For this review, take the finished solid that the model builds, in its own axes (mm). A direction names the side the tool comes from. Round coordinates to 2 decimals unless told otherwise and drop trailing zeros. Order: outer loops, then holes, each group sorted by start corner. A loop starts at its lowest first (then second) coordinate and runs counter-clockwise, first axis right, second up. Notation, with made-up numbers: M 78.5,9 L 119.5,9 A33 ccw 119.5,42 Z; hole C 17,46 d4. An arc over 180 degrees is marked long. Answer as a JSON object with one key per item and string values.
from build123d import *

# Parameters (mm, degrees)
AUFSATZ_LINEAR_AUSTRAGEN2_DEPTH = 14
SKIZZE3_W                       = 10.8
SKIZZE3_H                       = 4
SKIZZE3_H_2                     = 8
SCHNITT_LINEAR_AUSTRAGEN1_DEPTH = 201.389926144
SCHNITT_LINEAR_AUSTRAGEN2_DEPTH = 202.674849696


with BuildPart() as part:
    # Skizze1 → Aufsatz-Linear austragen2 (new, symmetric)
    with BuildSketch(Plane.XY):
        with BuildLine():
            Line((-198.15, 0), (-198.15, -2))
            Line((-198.15, -2), (-199.65, -2))
            Line((-199.65, -2), (-199.65, 0))
            ThreePointArc((-199.65, 0), (-198.288046533, 3.288046533), (-195, 4.65))
            Line((-195, 4.65), (195, 4.65))
            ThreePointArc((195, 4.65), (198.288046533, 3.288046533), (199.65, 0))
            Line((199.65, 0), (199.65, -2))
            Line((199.65, -2), (198.15, -2))
            Line((198.15, -2), (198.15, 0))
            ThreePointArc((198.15, 0), (195, 3.15), (191.85, 0))
            Line((191.85, 0), (191.85, -2))
            Line((191.85, -2), (188.85, -2))
            Line((188.85, -2), (188.85, -5.35))
            Line((188.85, -5.35), (-188.85, -5.35))
            Line((-188.85, -5.35), (-188.85, -2))
            Line((-188.85, -2), (-191.85, -2))
            Line((-191.85, -2), (-191.85, 0))
            ThreePointArc((-191.85, 0), (-195, 3.15), (-198.15, 0))
        make_face()
    extrude(amount=AUFSATZ_LINEAR_AUSTRAGEN2_DEPTH, both=True)

    # Skizze3 → Schnitt-Linear austragen1 (cut, through all)
    with BuildSketch(Plane.XZ.offset(5.35)):
        with Locations((-194.25, 12)):
            Rectangle(SKIZZE3_W, SKIZZE3_H)
        with Locations((-194.25, 2)):
            Rectangle(SKIZZE3_W, SKIZZE3_H_2)
        with Locations((-194.25, -10)):
            Rectangle(SKIZZE3_W, SKIZZE3_H_2)
        with Locations((194.25, 10)):
            Rectangle(SKIZZE3_W, SKIZZE3_H_2)
        with Locations((194.25, -2)):
            Rectangle(SKIZZE3_W, SKIZZE3_H_2)
        with Locations((194.25, -12)):
            Rectangle(SKIZZE3_W, SKIZZE3_H)
    extrude(amount=-SCHNITT_LINEAR_AUSTRAGEN1_DEPTH, mode=Mode.SUBTRACT)

    # Skizze4 → Schnitt-Linear austragen2 (cut, through all)
    with BuildSketch(Plane.XY.offset(14)):
        Polygon((174.5, 4.65), (174.5, 3.15), (184.5, 3.15), (184.5, -5.35), (-199.65, -5.35), (-199.65, 4.65), align=None)
    extrude(amount=-SCHNITT_LINEAR_AUSTRAGEN2_DEPTH, mode=Mode.SUBTRACT)


solid = part.part
1) Add section D-D on x = 182. State the section outline as (y, z) points, and give its area (3 significant figures).
Geometry check:
{"outline": "M 3.15,-14 L 4.65,-14 L 4.65,14 L 3.15,14 Z", "area": "42.0 mm²"}
2) For L1, parallel to Z at x = 197, y = 3; L2, parallel to X at y = -1.75, z = 2.5; L3, parallel to X at y = 0, z = 1.75, list the stretches that pass through material, from the lowest coordinate up.
Geometry check:
{"L1": "z = -10 to -6, 2 to 6", "L2": "x = 184.5 to 191.85, 198.15 to 199.65", "L3": "x = 184.5 to 188.85"}
3) Mouldability with a two-part tool opening along X and no side actions: class faces 4 (the cylindrical face through (195.07, 3.15, -7.97)), 5 (the cylindrical face through (198.252, 3.324, 4.028)), 6 (the flat face through (182, 4.65, 0)) as +X half, -X half, draft (parallel to the pull), parting line (faces both ways), or undercut.
Geometry check:
{"face 4": "undercut", "face 5": "+X half", "face 6": "draft"}
4) Machinability: for faces 1 (the flat face through (199, -2, -8)), 2 (the flat face through (198.15, -1, -8)), 3 (the flat face through (193, 3, 6)), which of the approach directions +Z, -Z, +X, -X, +Y, -Y give a long, thin tool a straight path to every point of the face, cutting with its end or side? Answer none if there is none.
Geometry check:
{"face 1": "+Z, -Z, +X, -Y", "face 2": "+Z, -Z, -Y", "face 3": "+Z, +X, +Y, -Y"}
5) Insertion check: P1, Ø6, axis at x = 180.5, z = -6.5, coming from the -Y side; P2, Ø11, axis at x = 180.5, z = -5.5, coming from the -Y side; P3, Ø2.5, axis at y = -2, z = 5, coming from the -X side; P4, Ø2, axis at x = 193.5, z = -6, coming from the -Y side. Each pin has a flat end and moves straight along its axis. Give the tip position at first contact, or say it passes through.
Geometry check:
{"P1": "stops at y = 3.15", "P2": "stops at y = -5.35", "P3": "stops at x = 184.5", "P4": "stops at y = 1.92"}
6) Add section B-B on y = -1.25. State the section outline as (x, z) points, and give its area (3 significant figures).
Geometry check:
{"outline": "M 184.5,-14 L 188.85,-14 L 188.85,-10 L 191.85,-10 L 191.85,-6 L 188.85,-6 L 188.85,2 L 191.85,2 L 191.85,6 L 188.85,6 L 188.85,14 L 184.5,14 Z; M 198.15,-10 L 199.65,-10 L 199.65,-6 L 198.15,-6 Z; M 198.15,2 L 199.65,2 L 199.65,6 L 198.15,6 Z", "area": "158 mm²"}
7) Add section A-A on x = 191.5. State the section outline as (y, z) points, and give its area (3 significant figures).
Geometry check:
{"outline": "M -2,-10 L 4.65,-10 L 4.65,-6 L -2,-6 Z; M -2,2 L 4.65,2 L 4.65,6 L -2,6 Z", "area": "53.2 mm²"}
8) Add section C-C on z = 11.5. State the section outline as (x, y) points.
Geometry check:
{"outline": "M 174.5,3.15 L 184.5,3.15 L 184.5,-5.35 L 188.85,-5.35 L 188.85,4.65 L 174.5,4.65 Z"}
